Source: CAD feature listing. Evaluate the final solid. Frame: model axes, mm. A direction names the side the tool comes from. Give positions to 0.01 mm unless a question says otherwise; leave off trailing zeros. Write each loop counter-clockwise with the first axis right and the second up, starting at its lowest first coordinate (ties: lowest second). Pieces come first, ordered by that corner, then holes. Notation, with made-up numbers: (53, -13.75) -> (58, -13.75) arc R32 ccw to (58, 19.25) -> close; hole circle Ø1 at (11.25, -25). An arc over 180 degrees is marked (long way). Write item = value, one per line.
from build123d import *

# Parameters (mm, degrees)
CUT_EXTRUDE1_DEPTH = 2.8


with BuildPart() as part:
    # Sketch2 → Revolve1 (revolve)
    with BuildSketch(Plane(origin=(0, 0, 0), x_dir=(0, 0, -1), z_dir=(1, 0, 0)), mode=Mode.PRIVATE) as revolve1_sk:
        with BuildLine():
            Line((-16.65, 0), (16.65, 0))
            Line((16.65, 0), (16.65, 2.2))
            Line((16.65, 2.2), (15.85, 3))
            Line((15.85, 3), (-13.35, 3))
            Line((-13.35, 3), (-13.35, 5.25))
            Line((-13.35, 5.25), (-13.845, 5.25))
            ThreePointArc((-13.845, 5.25), (-15.433520981, 4.356906156), (-16.65, 3))
            Line((-16.65, 3), (-16.65, 0))
        make_face()
    revolve(revolve1_sk.sketch.rotate(Axis((0, 0, 16.65), (0, 0, -1)), 90), axis=Axis((0, 0, 16.65), (0, 0, -1)))

    # Sketch3 → Cut-Extrude1 (cut)
    with BuildSketch(Plane.XY.offset(16.65)):
        Polygon((0, 2.309401077), (-2, 1.154700538), (-2, -1.154700538), (0, -2.309401077), (2, -1.154700538), (2, 1.154700538), align=None)
    extrude(amount=-CUT_EXTRUDE1_DEPTH, mode=Mode.SUBTRACT)

    # Cut-Extrude2 cone 1 section (through the dimple's axis) → Cut-Extrude2 (revolve, cut)
    with BuildSketch(Plane(origin=(0, 0, 16.65), x_dir=(0, -1, 0), z_dir=(1, 0, 0))):
        Polygon((0, 0), (2.309401077, 0), (0, 2.309401077), align=None)
    revolve(axis=Axis((0, 0, 16.65), (0, 0, -1)), mode=Mode.SUBTRACT)


solid = part.part
(1) Pull-direction query (Y, two-part tool) for faces 4 (the face through (0.99, -1.74, 15.27)), 5 (the face through (0, 0, 13.85)), 6 (the face through (-2.3, 2.3, 13.35)), 7 (the face through (5, -1.6, 13.6)); classes: pulls with the +Y half, pulls with the -Y half, needs draft (parallel to the pull), parting line crosses it, or undercut.
Values follow:
face_4 = undercut
face_5 = undercut
face_6 = needs draft
face_7 = parting line crosses it
(2) Material intervals for line 1 (Z direction, x = -1.5, y = -1); line 2 (Z direction, x = -3.25, y = 0.75); line 3 (Y direction, x = 3.5, z = 14), sorted ascending.
Values follow:
line_1 = -16.65 to 13.85
line_2 = 13.35 to 16.42
line_3 = -3.83 to 3.83
(3) Section query B-B (z = -9.5). Return loops of the section in (x, y).
Values follow:
outline = circle Ø6 at (0, 0)
(4) Section query C-C (z = 14.5). Return loops of the section in (x, y), plus the area to 3 significant figures.
Values follow:
outline = circle Ø9.93 at (0, 0); hole (-2, -1.15) -> (0, -2.31) -> (2, -1.15) -> (2, 1.15) -> (0, 2.31) -> (-2, 1.15) -> close
area = 63.5 mm2
(5) Access query for faces 1 (the face through (2.86, -0.9, -1.05)), 2 (the face through (0, 0, -16.65)), 3 (the face through (-1.09, 1.856, 16.493)). Directions: +Z, -Z, +X, -X, +Y, -Y. A direction counts if a zero-diameter tool reaches every point of the face in a straight line with its end or side. Return the directions, or none.
Values follow:
face_1 = -Z
face_2 = -Z, +X, -X, +Y, -Y
face_3 = +Z
(6) Section query A-A (y = 0). Return loops of the section in (x, z) (3 decimals), plus the area to 3 significant figures.
Values follow:
outline = (-5.25, 13.35) -> (-3, 13.35) -> (-3, -15.85) -> (-2.2, -16.65) -> (2.2, -16.65) -> (3, -15.85) -> (3, 13.35) -> (5.25, 13.35) -> (5.25, 13.845) arc R5.585 ccw to (3, 16.65) -> (2.309, 16.65) -> (2, 16.341) -> (2, 13.85) -> (-2, 13.85) -> (-2, 16.341) -> (-2.309, 16.65) -> (-3, 16.65) arc R5.585 ccw to (-5.25, 13.845) -> close
area = 198 mm2
(7) First-contact query: pin 1 (1.8 mm diameter, centred on y = 0, z = 15.5, fed in from -X); pin 2 (5 mm diameter, centred on y = 3.5, z = 7.5, fed in from -X); pin 3 (4 mm diameter, centred on x = -1, z = -6.5, fed in from -Y). Flat tips, straight axial feed; report the tip coordinate or a pass-through.
Values follow:
pin_1 = -4.91
pin_2 = -2.83
pin_3 = -3
